Design review of the part built by this model. Coordinates are the model's own, in mm. Face numbers are marked on the shaded views. Coordinates: 2 decimals unless noted, no trailing zeros. Order: outer loops, then holes, each group sorted by start corner. A loop starts at its lowest first (then second) coordinate and runs counter-clockwise, first axis right, second up. Notation, with made-up numbers: (60, -35.75) -> (69, -35.75) arc R16 ccw to (69, -10.75) -> close; hole circle Ø5 at (-17.75, -21.5). An arc over 180 degrees is marked (long way). Use a Markdown table: item, result. Add a question column.
Q1. Wall thickness on probe 1 along Y at (x, z) = (-6.25, 20); probe 2 along X at (y, z) = (15, 7.5); probe 3 along Z at (x, y) = (-22, 11): over which ranges is each line inside the solid? List them lowest first.
Q2. Add section A-A (y = 12.5). State the section outline as (x, z) points.
Q3. Insertion check: pin 1 (2.5 mm diameter, centred on x = -20.5, y = 11, fed in from -Z); pin 2 (1.5 mm diameter, centred on x = -13.5, y = 10, fed in from -Z). Each pin has a flat end and moves straight along its axis. Give the tip position at first contact, or say it passes through.
Q4. Add section B-B (z = 31.5). State the section outline as (x, y) points, then the cut area to 3 significant figures.
Q5. Add section D-D (x = -13.5). State the section outline as (y, z) points, then the cut area to 3 significant figures.
Q6. Add section C-C (x = -3.25). State the section outline as (y, z) points.
Q7. The part is to be moulded in two halves that separate along Y. For the marked faces 1, 2, 3 and 4, say which applies: pulls with the +Y half, pulls with the -Y half, needs draft (parallel to the pull), parting line crosses it, or undercut.
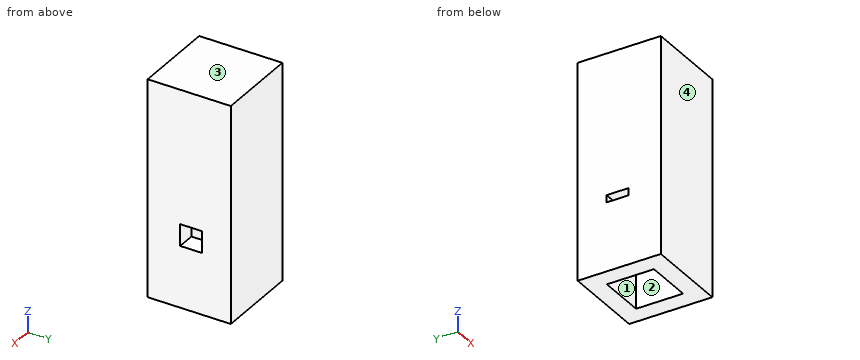
from build123d import *

# Parameters (mm, degrees)
SKETCH_3_W          = 23
SKETCH_3_H          = 23
SKETCH_3_W_2        = 13
SKETCH_3_H_2        = 13
EXTRUDE_1_DEPTH     = 33
SKETCH_6_W          = 23
SKETCH_6_H          = 23
EXTRUDE_3_DEPTH     = 27
SKETCH_9_W          = 6
SKETCH_9_H          = 6
EXTRUDE_5_DEPTH     = 5
SKETCH_9_2_W        = 6
SKETCH_9_2_H        = 6
CUT_EXTRUDE_3_DEPTH = 5
SKETCH_10_W         = 2
SKETCH_10_H         = 6
CUT_EXTRUDE_4_DEPTH = 5


with BuildPart() as part:
    # 草图3 → 凸台-拉伸1 (new body)
    with BuildSketch(Plane.XY):
        with Locations((-11.5, 11.5)):
            Rectangle(SKETCH_3_W, SKETCH_3_H)
        with Locations((-11.5, 11.5)):
            Rectangle(SKETCH_3_W_2, SKETCH_3_H_2, mode=Mode.SUBTRACT)
    extrude(amount=EXTRUDE_1_DEPTH)

    # 草图6 → 凸台-拉伸3 (add)
    with BuildSketch(Plane.XY.offset(33)):
        with Locations((-11.5, 11.5)):
            Rectangle(SKETCH_6_W, SKETCH_6_H)
    extrude(amount=EXTRUDE_3_DEPTH)

    # 草图9 → 凸台-拉伸5 (add)
    with BuildSketch(Plane(origin=(0, 0, 0), x_dir=(0, 0, -1), z_dir=(1, 0, 0))):
        with Locations((-20, 12)):
            Rectangle(SKETCH_9_W, SKETCH_9_H)
    extrude(amount=-EXTRUDE_5_DEPTH)

    # 草图9<2> → 切除-拉伸3 (cut)
    with BuildSketch(Plane(origin=(0, 0, 0), x_dir=(0, 0, -1), z_dir=(1, 0, 0))):
        with Locations((-20, 12)):
            Rectangle(SKETCH_9_2_W, SKETCH_9_2_H)
    extrude(amount=-CUT_EXTRUDE_3_DEPTH, mode=Mode.SUBTRACT)

    # 草图10 → 切除-拉伸4 (cut)
    with BuildSketch(Plane.ZY.offset(23)):
        with Locations((20, 12)):
            Rectangle(SKETCH_10_W, SKETCH_10_H)
    extrude(amount=-CUT_EXTRUDE_4_DEPTH, mode=Mode.SUBTRACT)


solid = part.part
Established:
| question | item | result |
|---|---|---|
| 1 | probe 1 | 0 to 5, 18 to 23 |
| 1 | probe 2 | -23 to -18, -5 to 0 |
| 1 | probe 3 | 0 to 19, 21 to 60 |
| 2 | outline | (-23, 0) -> (-18, 0) -> (-18, 19) -> (-23, 19) -> close; (-23, 21) -> (-18, 21) -> (-18, 33) -> (-5, 33) -> (-5, 23) -> (0, 23) -> (0, 60) -> (-23, 60) -> close; (-5, 0) -> (0, 0) -> (0, 17) -> (-5, 17) -> close |
| 3 | pin 1 | z = 0 |
| 3 | pin 2 | z = 33 |
| 4 | outline | (-23, 0) -> (0, 0) -> (0, 23) -> (-23, 23) -> close; hole (-18, 5) -> (-5, 5) -> (-5, 18) -> (-18, 18) -> close |
| 4 | area | 360 mm^2 |
| 5 | outline | (0, 0) -> (5, 0) -> (5, 33) -> (18, 33) -> (18, 0) -> (23, 0) -> (23, 60) -> (0, 60) -> close |
| 5 | area | 951 mm^2 |
| 6 | outline | (0, 0) -> (23, 0) -> (23, 60) -> (0, 60) -> close; hole (9, 17) -> (15, 17) -> (15, 23) -> (9, 23) -> close |
| 7 | face 1 | undercut |
| 7 | face 2 | undercut |
| 7 | face 3 | needs draft |
| 7 | face 4 | pulls with the -Y half |
